```python
from build123d import *

# Parameters (mm, degrees)
SKETCH1_W           = 69.85
SKETCH1_H           = 110
SKETCH1_R           = 19.5
SKETCH1_R_2         = 3.25755
SKETCH1_R_3         = 1.45
BOSS_EXTRUDE1_DEPTH = 5


with BuildPart() as part:
    # Sketch1 → Boss-Extrude1 (new body)
    with BuildSketch(Plane.YZ):
        Rectangle(SKETCH1_W, SKETCH1_H)
        with Locations((0, 19.75)):
            Circle(SKETCH1_R, mode=Mode.SUBTRACT)
        with Locations((-25, -42.3)):
            Circle(SKETCH1_R_2, mode=Mode.SUBTRACT)
        with Locations((25, -42.3)):
            Circle(SKETCH1_R_2, mode=Mode.SUBTRACT)
        with Locations((-20.56810334, 7.875)):
            Circle(SKETCH1_R_3, mode=Mode.SUBTRACT)
        with Locations((20.56810334, 7.875)):
            Circle(SKETCH1_R_3, mode=Mode.SUBTRACT)
        with Locations((0, 43.5)):
            Circle(SKETCH1_R_3, mode=Mode.SUBTRACT)
    extrude(amount=BOSS_EXTRUDE1_DEPTH)


solid = part.part
```
The listing builds one solid part. Answer for the finished solid, in the listing's coordinates (mm). Coordinates: 2 decimals unless noted, no trailing zeros. Loops run counter-clockwise (first coordinate to the right, second up) from the corner with the lowest first, then second, coordinate; pieces in that order, holes last. Notation, with made-up numbers: (-28, -15.75) -> (9, -15.75) arc R12 ccw to (9, -4.75) -> close; hole circle Ø3 at (64, 80). An arc over 180 degrees is marked (long way). Return JSON: item names as keys, results as strings. Group by question number.
(1) A cutting plane is placed at B-B on y = -25. Write down the section's boundary in (x, z), and give its area (3 significant figures).
(2) A cutting plane is placed at D-D on y = 0. Write down the section's boundary in (x, z), and give its area (4 significant figures).
(3) Determine the mould class of faces 1 (the cylindrical face through (2.5, 21.9, 7.3)), 2 (the flat face through (2, -34.925, -1)), 3 (the flat face through (2, 0, -55)), 4 (the flat face through (2, 34.925, -1)) for opening direction Y: released by +Y, released by -Y, zero draft, split by the parting line, or undercut.
(4) Find the intervals of material crossed by probe 1 along Z at (x, y) = (2.8, 25); probe 2 along Y at (x, z) = (2.95, -44) (3 decimals); probe 3 along Y at (x, z) = (2.05, 16) (3 decimals), in increasing order. Write a range as from..to.
(5) A cutting plane is placed at A-A on z = 43.5. Write down the section's boundary in (x, y) (3 decimals).
(6) Given pin 1 Ø4 at (y, z) = (-25, -42.3) entering from +X, flat-ended and moving along its own axis, determine where the tip first touches the part or whether it passes through.
(7) A cutting plane is placed at C-C on z = -42.3. Write down the section's boundary in (x, y) (3 decimals).
The answers:
{
 "1": {"outline": "(0, -55) -> (5, -55) -> (5, -45.56) -> (0, -45.56) -> close; (0, -39.04) -> (5, -39.04) -> (5, 55) -> (0, 55) -> close", "area": "517 mm^2"},
 "2": {"outline": "(0, -55) -> (5, -55) -> (5, 0.25) -> (0, 0.25) -> close; (0, 39.25) -> (5, 39.25) -> (5, 42.05) -> (0, 42.05) -> close; (0, 44.95) -> (5, 44.95) -> (5, 55) -> (0, 55) -> close", "area": "340.5 mm^2"},
 "3": {"face 1": "undercut", "face 2": "released by -Y", "face 3": "zero draft", "face 4": "released by +Y"},
 "4": {"probe 1": "z = -55..-45.56, -39.04..55", "probe 2": "y = -34.925..-27.779, -22.221..22.221, 27.779..34.925", "probe 3": "y = -34.925..-19.136, 19.136..34.925"},
 "5": {"outline": "(0, -34.925) -> (5, -34.925) -> (5, -1.45) -> (0, -1.45) -> close; (0, 1.45) -> (5, 1.45) -> (5, 34.925) -> (0, 34.925) -> close"},
 "6": {"pin 1": "passes through"},
 "7": {"outline": "(0, -34.925) -> (5, -34.925) -> (5, -28.258) -> (0, -28.258) -> close; (0, -21.742) -> (5, -21.742) -> (5, 21.742) -> (0, 21.742) -> close; (0, 28.258) -> (5, 28.258) -> (5, 34.925) -> (0, 34.925) -> close"}
}
